Can you work these out from the model? Positions are in its coordinate system, mm. A direction names the side the tool comes from. Give positions to 0.01 mm unless a question says otherwise; leave off trailing zeros. Write each loop counter-clockwise with the first axis right and the second up, starting at its lowest first coordinate (ties: lowest second). Pieces come first, ordered by that corner, then holes.
1. If I drill on probe 1 along X at (y, z) = (17.5, 2); probe 2 along X at (y, z) = (30, 4.75); probe 3 along Y at (x, z) = (-59, 4.05), over which ranges is the centre line in solid material (lowest first)?
2. On a 3-axis mill with a long thin cutter (end or side, diameter ignored), from which of +Z, -Z, +X, -X, +Y, -Y can I reach the whole of each face in a straight line? I mean faces 4 (the flat face through (115, 17, 3)), 5 (the flat face through (1.82, -29.877, 2.958)). Say none if no direction works.
3. Thinking about a two-plate mould opening in X: for faces 1 (the flat face through (-115, 17, 3)), 2 (the flat face through (-1.8, 5.6, 6)), 3 (the flat face through (109, 20, 3)), which applies, pulls with the +X half, pulls with the -X half, needs draft (parallel to the pull), parting line crosses it, or undercut?
4. Suppose I cut it at A-A (x = -45). Please give me the cut outline in (y, z).
5. I'm going to push flat-ended pins straight in: pin 1 (2.5 mm diameter, centred on x = -81, y = -14, fed in from -Z); pin 2 (5 mm diameter, centred on x = 59, y = -9, fed in from -Z); pin 3 (3.5 mm diameter, centred on x = 59, y = 9, fed in from -Z). Where does each tip first touch, or does it pass through?
```python
from build123d import *

# Parameters (mm, degrees)
SKETCH_1_W          = 260
SKETCH_1_H          = 70
EXTRUDE_1_DEPTH     = 6
CUT_EXTRUDE_1_DEPTH = 260
SKETCH_3_R          = 1.5
CUT_EXTRUDE_2_DEPTH = 10
SKETCH_4_R          = 1.5
CUT_EXTRUDE_3_DEPTH = 10
SKETCH_5_R          = 1.5
CUT_EXTRUDE_4_DEPTH = 33
SKETCH_6_R          = 1.5
SKETCH_6_W          = 12
SKETCH_6_H          = 6
CUT_EXTRUDE_5_DEPTH = 10
SKETCH_7_R          = 1.5
CUT_EXTRUDE_6_DEPTH = 10
CHAMFER_1_SIZE      = 2
CHAMFER_2_SIZE      = 2
CHAMFER_3_SIZE      = 2
CHAMFER_4_SIZE      = 2


with BuildPart() as part:
    # 草图1 → 凸台-拉伸1 (new body)
    with BuildSketch(Plane.XY):
        Rectangle(SKETCH_1_W, SKETCH_1_H)
    extrude(amount=EXTRUDE_1_DEPTH)

    # 草图2 → 切除-拉伸1 (cut)
    with BuildSketch(Plane(origin=(130, 0, 0), x_dir=(0, 0, -1), z_dir=(1, 0, 0))):
        Polygon((0, -35), (-6, -24.607695155), (-6, -35), align=None)
    extrude(amount=-CUT_EXTRUDE_1_DEPTH, mode=Mode.SUBTRACT)

    # 草图3 → 切除-拉伸2 (cut)
    with BuildSketch(Plane.XY.offset(6)):
        with Locations((-59, 9)):
            Circle(SKETCH_3_R)
        with Locations((59, 9)):
            Circle(SKETCH_3_R)
    extrude(amount=-CUT_EXTRUDE_2_DEPTH, mode=Mode.SUBTRACT)

    # 草图4 → 切除-拉伸3 (cut)
    with BuildSketch(Plane(origin=(0, 0, 0), x_dir=(-1, 0, 0), z_dir=(0, 0, -1))):
        with Locations((-59, 27)):
            Circle(SKETCH_4_R)
        with Locations((-59, -9)):
            Circle(SKETCH_4_R)
        with Locations((59, 27)):
            Circle(SKETCH_4_R)
        with Locations((59, -9)):
            Circle(SKETCH_4_R)
    extrude(amount=-CUT_EXTRUDE_3_DEPTH, mode=Mode.SUBTRACT)

    # 草图5 → 切除-拉伸4 (cut)
    with BuildSketch(Plane.XY.offset(6)):
        with Locations((0, 27)):
            Circle(SKETCH_5_R)
        with Locations((0, 9)):
            Circle(SKETCH_5_R)
        with Locations((0, -9)):
            Circle(SKETCH_5_R)
    extrude(amount=-CUT_EXTRUDE_4_DEPTH, mode=Mode.SUBTRACT)

    # 草图6 → 切除-拉伸5 (cut)
    with BuildSketch(Plane.XY.offset(6)):
        with Locations((-99, 20)):
            Circle(SKETCH_6_R)
        with Locations((-115, 20)):
            Rectangle(SKETCH_6_W, SKETCH_6_H)
    cut_extrude_5 = extrude(amount=-CUT_EXTRUDE_5_DEPTH, mode=Mode.SUBTRACT)

    # 镜向1: 切除-拉伸5 across plane
    add(cut_extrude_5.mirror(Plane(origin=(0, 0, 0), x_dir=(0, 0, 1), z_dir=(1, 0, 0))), mode=Mode.SUBTRACT)

    # 草图7 → 切除-拉伸6 (cut)
    with BuildSketch(Plane.XY.offset(6)):
        with Locations((-126, 32)):
            Circle(SKETCH_7_R)
        with Locations((-81, 32)):
            Circle(SKETCH_7_R)
        with Locations((-81, -14)):
            Circle(SKETCH_7_R)
        with Locations((-126, -14)):
            Circle(SKETCH_7_R)
    cut_extrude_6 = extrude(amount=-CUT_EXTRUDE_6_DEPTH, mode=Mode.SUBTRACT)

    # 镜向2: 切除-拉伸6 across plane
    add(cut_extrude_6.mirror(Plane(origin=(0, 0, 0), x_dir=(0, 0, 1), z_dir=(1, 0, 0))), mode=Mode.SUBTRACT)

    # 倒角1
    # the kernel refuses this chamfer: 2 mm, written as the material it takes off along each edge
    with BuildSketch(Plane(origin=(126, 32, 0), x_dir=(-1, 0, 0), z_dir=(0, 1, 0))) as chamfer_1_piece_1:
        Polygon((1.5 + CHAMFER_1_SIZE, 0), (1.5, CHAMFER_1_SIZE), (1.5, 0), align=None)
    revolve(axis=Axis((126, 32, 0), (0, 0, 1)), mode=Mode.SUBTRACT)

    # 倒角2
    # the kernel refuses this chamfer: 2 mm, written as the material it takes off along each edge
    with BuildSketch(Plane(origin=(-126, 32, 0), x_dir=(1, 0, 0), z_dir=(0, -1, 0))) as chamfer_2_piece_1:
        Polygon((1.5 + CHAMFER_2_SIZE, 0), (1.5, CHAMFER_2_SIZE), (1.5, 0), align=None)
    revolve(axis=Axis((-126, 32, 0), (0, 0, 1)), mode=Mode.SUBTRACT)
    with BuildSketch(Plane(origin=(-126, 32, 6), x_dir=(1, 0, 0), z_dir=(0, -1, 0))) as chamfer_2_piece_2:
        Polygon((1.5 + CHAMFER_2_SIZE, 0), (1.5, -CHAMFER_2_SIZE), (1.5, 0), align=None)
    revolve(axis=Axis((-126, 32, 6), (0, 0, 1)), mode=Mode.SUBTRACT)
    with BuildSketch(Plane(origin=(-81, 32, 0), x_dir=(1, 0, 0), z_dir=(0, -1, 0))) as chamfer_2_piece_3:
        Polygon((1.5 + CHAMFER_2_SIZE, 0), (1.5, CHAMFER_2_SIZE), (1.5, 0), align=None)
    revolve(axis=Axis((-81, 32, 0), (0, 0, 1)), mode=Mode.SUBTRACT)
    with BuildSketch(Plane(origin=(-81, 32, 6), x_dir=(1, 0, 0), z_dir=(0, -1, 0))) as chamfer_2_piece_4:
        Polygon((1.5 + CHAMFER_2_SIZE, 0), (1.5, -CHAMFER_2_SIZE), (1.5, 0), align=None)
    revolve(axis=Axis((-81, 32, 6), (0, 0, 1)), mode=Mode.SUBTRACT)
    with BuildSketch(Plane(origin=(81, 32, 0), x_dir=(-1, 0, 0), z_dir=(0, 1, 0))) as chamfer_2_piece_5:
        Polygon((1.5 + CHAMFER_2_SIZE, 0), (1.5, CHAMFER_2_SIZE), (1.5, 0), align=None)
    revolve(axis=Axis((81, 32, 0), (0, 0, 1)), mode=Mode.SUBTRACT)
    with BuildSketch(Plane(origin=(59, 27, 0), x_dir=(-1, 0, 0), z_dir=(0, -1, 0))) as chamfer_2_piece_6:
        Polygon((1.5 + CHAMFER_2_SIZE, 0), (1.5, -CHAMFER_2_SIZE), (1.5, 0), align=None)
    revolve(axis=Axis((59, 27, 0), (0, 0, -1)), mode=Mode.SUBTRACT)
    with BuildSketch(Plane(origin=(-59, 27, 0), x_dir=(-1, 0, 0), z_dir=(0, -1, 0))) as chamfer_2_piece_7:
        Polygon((1.5 + CHAMFER_2_SIZE, 0), (1.5, -CHAMFER_2_SIZE), (1.5, 0), align=None)
    revolve(axis=Axis((-59, 27, 0), (0, 0, -1)), mode=Mode.SUBTRACT)
    with BuildSketch(Plane(origin=(0, 27, 6), x_dir=(1, 0, 0), z_dir=(0, -1, 0))) as chamfer_2_piece_8:
        Polygon((1.5 + CHAMFER_2_SIZE, 0), (1.5, -CHAMFER_2_SIZE), (1.5, 0), align=None)
    revolve(axis=Axis((0, 27, 6), (0, 0, 1)), mode=Mode.SUBTRACT)

    # 倒角3
    chamfer_3_edges = [part.edges().sort_by_distance(p)[0] for p in [
        (-82.5, -14, 0),
        (-127.5, -14, 0),
        (-60.5, 9, 0),
        (57.5, 9, 0),
        (-57.5, -9, 0),
        (-1.5, 27, 0),
        (-1.5, 9, 0),
        (-1.5, 9, 6),
        (-1.5, -9, 0),
        (-100.5, 20, 0),
        (100.5, 20, 0),
    ]]
    chamfer(chamfer_3_edges, length=CHAMFER_3_SIZE)

    # 倒角4
    chamfer_4_edges = [part.edges().sort_by_distance(p)[0] for p in [
        (82.5, -14, 0),
        (127.5, -14, 0),
        (60.5, -9, 0),
    ]]
    chamfer(chamfer_4_edges, length=CHAMFER_4_SIZE)


solid = part.part
```
Checks:
1. probe 1: x = -130 to -121, -109 to 109, 121 to 130
1. probe 2: x = -130 to -127.03, -124.97 to -82.03, -79.97 to 130
1. probe 3: y = -27.99 to -10.5, -7.5 to 7.5, 10.5 to 25.5, 28.5 to 35
2. face 4: +Z, -Z
2. face 5: +Z, +X, -X, -Y
3. face 1: undercut
3. face 2: needs draft
3. face 3: undercut
4. outline: (-35, 0) - (35, 0) - (35, 6) - (-24.61, 6) - close
5. pin 1: passes through
5. pin 2: stops at z = 1
5. pin 3: stops at z = 1.75
